```python
from build123d import *

# Parameters (mm, degrees)
SKETCH_1_R      = 20
SKETCH_1_R_2    = 2.55
EXTRUDE_2_DEPTH = 4
FILLET_1_R      = 3


with BuildPart() as part:
    # Эскиз1 → Бобышка-Вытянуть2 (new body)
    with BuildSketch(Plane.XY):
        Polygon((-40, 0), (40, 0), (40, -53.2), (30, -53.2), (30, -57.2), (5, -57.2), (5, -53.2), (-5, -53.2), (-5, -57.2), (-30, -57.2), (-30, -53.2), (-40, -53.2), align=None)
        with Locations((0, -28.2)):
            Circle(SKETCH_1_R, mode=Mode.SUBTRACT)
        with Locations((-23.57, -4.63)):
            Circle(SKETCH_1_R_2, mode=Mode.SUBTRACT)
        with Locations((23.57, -4.63)):
            Circle(SKETCH_1_R_2, mode=Mode.SUBTRACT)
        with Locations((23.57, -51.77)):
            Circle(SKETCH_1_R_2, mode=Mode.SUBTRACT)
        with Locations((-23.57, -51.77)):
            Circle(SKETCH_1_R_2, mode=Mode.SUBTRACT)
    extrude(amount=EXTRUDE_2_DEPTH)

    # Скругление1
    fillet_1_edges = [part.edges().sort_by_distance(p)[0] for p in [
        (-40, 0, 2),
        (40, 0, 2),
    ]]
    fillet(fillet_1_edges, radius=FILLET_1_R)


solid = part.part
```
For this review, take the finished solid that the model builds, in its own axes (mm). A direction names the side the tool comes from. Give positions to 0.01 mm unless a question says otherwise; leave off trailing zeros. Write each loop counter-clockwise with the first axis right and the second up, starting at its lowest first coordinate (ties: lowest second). Pieces come first, ordered by that corner, then holes.
Item 1: Insertion check: P1, Ø2, axis at y = -55.5, z = 2, coming from the +X side; P2, Ø2, axis at x = -37, z = 1.5, coming from the -Y side. Each pin has a flat end and moves straight along its axis. Give the tip position at first contact, or say it passes through.
Item 2: Machinability: for faces 1 (the face through (39.1, -0.86, 2.03)), 2 (the face through (-30, -55, 2)), 3 (the face through (35, -53.2, 2)), 4 (the face through (-5, -55, 2)), which of the approach directions +Z, -Z, +X, -X, +Y, -Y give a long, thin tool a straight path to every point of the face, cutting with its end or side? Answer none if there is none.
Item 3: Take a section at D-D (x = 0). Give the boundary of the cut face in (y, z), and give its area (3 significant figures).
Item 4: Take a section at B-B (x = -23.57). Give the boundary of the cut face in (y, z).
Item 5: Take a section at A-A (y = -28.2). Give the boundary of the cut face in (x, z), and give its area (3 significant figures).
Item 6: Take a section at C-C (z = 2.75). Give the boundary of the cut face in (x, y).
Item 7: The part is to be moulded in two halves that separate along X. For faces 5 (the face through (30, -55, 2)), 6 (the face through (23.24, -49.24, 1.97)), 7 (the face through (9, -9, 0)), 8 (the face through (-21.14, -3.86, 1.97)), say which applies: +X half, -X half, draft (parallel to the pull), parting line (faces both ways), or undercut.
Item 8: Wall thickness on probe 1 along Y at (x, z) = (-23.57, 1.4); probe 2 along Y at (x, z) = (0, 1.15); probe 3 along Y at (x, z) = (23, 0.4): over which ranges is each line inside the solid? List them lowest first.
Established:
1. P1: stops at x = 30
1. P2: stops at y = -53.2
2. face 1: +Z, -Z, +X, +Y
2. face 2: +Z, -Z, -X, -Y
2. face 3: +Z, -Z, +X, -Y
2. face 4: +Z, -Z, -Y
3. outline: (-53.2, 0) - (-48.2, 0) - (-48.2, 4) - (-53.2, 4) - close; (-8.2, 0) - (0, 0) - (0, 4) - (-8.2, 4) - close
3. area: 52.8 mm2
4. outline: (-57.2, 0) - (-54.32, 0) - (-54.32, 4) - (-57.2, 4) - close; (-49.22, 0) - (-7.18, 0) - (-7.18, 4) - (-49.22, 4) - close; (-2.08, 0) - (0, 0) - (0, 4) - (-2.08, 4) - close
5. outline: (-40, 0) - (-20, 0) - (-20, 4) - (-40, 4) - close; (20, 0) - (40, 0) - (40, 4) - (20, 4) - close
5. area: 160 mm2
6. outline: (-40, -53.2) - (-30, -53.2) - (-30, -57.2) - (-5, -57.2) - (-5, -53.2) - (5, -53.2) - (5, -57.2) - (30, -57.2) - (30, -53.2) - (40, -53.2) - (40, -3) arc R3 ccw to (37, 0) - (-37, 0) arc R3 ccw to (-40, -3) - close; hole circle Ø5.1 at (-23.57, -51.77); hole circle Ø5.1 at (-23.57, -4.63); hole circle Ø40 at (0, -28.2); hole circle Ø5.1 at (23.57, -51.77); hole circle Ø5.1 at (23.57, -4.63)
7. face 5: +X half
7. face 6: undercut
7. face 7: draft
7. face 8: undercut
8. probe 1: y = -57.2 to -54.32, -49.22 to -7.18, -2.08 to 0
8. probe 2: y = -53.2 to -48.2, -8.2 to 0
8. probe 3: y = -57.2 to -54.26, -49.28 to -7.12, -2.14 to 0
